```python
from build123d import *

# Parameters (mm, degrees)
F0_W     = 2082.8
F0_H     = 609.6
F1_DEPTH = 19.05
F2_R     = 12.7
F3_DEPTH = 25.4
F5_DEPTH = 6.35


with BuildPart() as f1:
    # F0 (on Top) → F1 (new body)
    with BuildSketch(Plane.XY):
        with Locations((1041.4, 304.8)):
            Rectangle(F0_W, F0_H)
    extrude(amount=F1_DEPTH)

    # F2 (on face) → F3 (cut)
    with BuildSketch(Plane.XY.offset(19.05)):
        with BuildLine():
            Line((1568.45, 584.2), (1435.1, 584.2))
            ThreePointArc((1435.1, 584.2), (1430.609872, 582.340128), (1428.75, 577.85))
            Line((1428.75, 577.85), (1428.75, 431.8))
            ThreePointArc((1428.75, 431.8), (1430.609872, 427.309872), (1435.1, 425.45))
            Line((1435.1, 425.45), (1568.45, 425.45))
            ThreePointArc((1568.45, 425.45), (1572.940128, 427.309872), (1574.8, 431.8))
            Line((1574.8, 431.8), (1574.8, 577.85))
            ThreePointArc((1574.8, 577.85), (1572.940128, 582.340128), (1568.45, 584.2))
        make_face()
        with BuildLine():
            Line((1136.65, 571.5), (946.15, 571.5))
            ThreePointArc((946.15, 571.5), (941.659872, 569.640128), (939.8, 565.15))
            Line((939.8, 565.15), (939.8, 501.65))
            ThreePointArc((939.8, 501.65), (941.659872, 497.159872), (946.15, 495.3))
            Line((946.15, 495.3), (1136.65, 495.3))
            ThreePointArc((1136.65, 495.3), (1141.140128, 497.159872), (1143, 501.65))
            Line((1143, 501.65), (1143, 565.15))
            ThreePointArc((1143, 565.15), (1141.140128, 569.640128), (1136.65, 571.5))
        make_face()
        with Locations((2082.8, 609.6)):
            Circle(F2_R)
    extrude(amount=-F3_DEPTH, mode=Mode.SUBTRACT)

    # F4 (on face) → F5 (cut)
    with BuildSketch(Plane.XY.offset(19.05)):
        with BuildLine():
            Line((1136.65, 584.2), (946.15, 584.2))
            ThreePointArc((946.15, 584.2), (932.679616, 578.620384), (927.1, 565.15))
            Line((927.1, 565.15), (927.1, 501.65))
            ThreePointArc((927.1, 501.65), (932.679616, 488.179616), (946.15, 482.6))
            Line((946.15, 482.6), (1136.65, 482.6))
            ThreePointArc((1136.65, 482.6), (1150.120384, 488.179616), (1155.7, 501.65))
            Line((1155.7, 501.65), (1155.7, 565.15))
            ThreePointArc((1155.7, 565.15), (1150.120384, 578.620384), (1136.65, 584.2))
        make_face()
        with BuildLine():
            ThreePointArc((1136.65, 571.5), (1141.140128, 569.640128), (1143, 565.15))
            Line((1143, 565.15), (1143, 501.65))
            ThreePointArc((1143, 501.65), (1141.140128, 497.159872), (1136.65, 495.3))
            Line((1136.65, 495.3), (946.15, 495.3))
            ThreePointArc((946.15, 495.3), (941.659872, 497.159872), (939.8, 501.65))
            Line((939.8, 501.65), (939.8, 565.15))
            ThreePointArc((939.8, 565.15), (941.659872, 569.640128), (946.15, 571.5))
            Line((946.15, 571.5), (1136.65, 571.5))
        make_face(mode=Mode.SUBTRACT)
    extrude(amount=-F5_DEPTH, mode=Mode.SUBTRACT)


solid = f1.part
```
Read the model definition and answer for the solid it produces. Units are mm, in the model's axes. Round coordinates to 2 decimals unless told otherwise and drop trailing zeros. Loops run counter-clockwise (first coordinate to the right, second up) from the corner with the lowest first, then second, coordinate; pieces in that order, holes last. Notation, with made-up numbers: (59.25, 46.25) -> (92.25, 46.25) arc R9 cw to (92.25, 51.25) -> close; hole circle Ø6 at (86.5, -28.5). An arc over 180 degrees is marked (long way). One line per item, written item: value.
1) The mould has two halves that part along Y. Classify faces 1 (the face through (1027, 309, 19.05)), 2 (the face through (1032, 492, 12.7)): pulls with the +Y half, pulls with the -Y half, needs draft (parallel to the pull), parting line crosses it, or undercut.
Answer list:
face 1: needs draft
face 2: undercut
2) A cutting plane is placed at A-A (x = 1116.5). Determine the outline of the cut face in (y, z).
Answer list:
outline: (0, 0) -> (495.3, 0) -> (495.3, 12.7) -> (482.6, 12.7) -> (482.6, 19.05) -> (0, 19.05) -> close; (571.5, 0) -> (609.6, 0) -> (609.6, 19.05) -> (584.2, 19.05) -> (584.2, 12.7) -> (571.5, 12.7) -> close
3) A cutting plane is placed at B-B (z = 7.25). Determine the outline of the cut face in (x, y), and give its area (3 significant figures).
Answer list:
outline: (0, 0) -> (2082.8, 0) -> (2082.8, 596.9) arc R12.7 cw to (2070.1, 609.6) -> (0, 609.6) -> close; hole (939.8, 501.65) arc R6.35 ccw to (946.15, 495.3) -> (1136.65, 495.3) arc R6.35 ccw to (1143, 501.65) -> (1143, 565.15) arc R6.35 ccw to (1136.65, 571.5) -> (946.15, 571.5) arc R6.35 ccw to (939.8, 565.15) -> close; hole (1428.75, 431.8) arc R6.35 ccw to (1435.1, 425.45) -> (1568.45, 425.45) arc R6.35 ccw to (1574.8, 431.8) -> (1574.8, 577.85) arc R6.35 ccw to (1568.45, 584.2) -> (1435.1, 584.2) arc R6.35 ccw to (1428.75, 577.85) -> close
area: 1,230,000 mm²
4) Consider L1, parallel to Y at x = 1077, z = 15.75; L2, parallel to Y at x = 963.5, z = 5.5. Determine where each line is inside the solid, lowest interval first. Write a range as [from, to].
Answer list:
L1: y = [0, 482.6], [584.2, 609.6]
L2: y = [0, 495.3], [571.5, 609.6]
